Here's how the part is built. I have some questions about the finished solid (model axes, mm). A direction names the side the tool comes from. Round coordinates to 2 decimals unless told otherwise and drop trailing zeros. Order: outer loops, then holes, each group sorted by start corner. A loop starts at its lowest first (then second) coordinate and runs counter-clockwise, first axis right, second up. Notation, with made-up numbers: (60.5, 41.25) -> (89.5, 41.25) arc R23 ccw to (89.5, 63.25) -> close; hole circle Ø11 at (5.5, 36.5). An arc over 180 degrees is marked (long way). Answer in a Markdown table with one row per item.
```python
from build123d import *

# Parameters (mm, degrees)
BOSS_EXTRUDE1_DEPTH     = 35
CUT_EXTRUDE3_DEPTH      = 84.964278119
CUT_EXTRUDE3_DEPTH_BACK = 84.964278119
SKETCH2_R               = 12.5
SKETCH2_R_2             = 15
CUT_EXTRUDE4_START      = 10
CUT_EXTRUDE4_DEPTH      = 25
CHAMFER1_SIZE           = 5


with BuildPart() as part:
    # Sketch1 → Boss-Extrude1 (new body)
    with BuildSketch(Plane(origin=(0, 0, 0), x_dir=(1, 0, 0), z_dir=(0, 1, 0))):
        with BuildLine():
            Line((-40, -16.905989232), (0, -40))
            Line((0, -40), (65, -40))
            Line((65, -40), (65, 20))
            Line((65, 20), (-4.844355629, 20))
            ThreePointArc((-4.844355629, 20), (-38.631222116, 27.900831925), (-40, -6.770509831))
            Line((-40, -6.770509831), (-40, -16.905989232))
        make_face()
    extrude(amount=BOSS_EXTRUDE1_DEPTH)

    # Sketch2 → Cut-Extrude3 (cut, two sides: drawn at the far end of the back side and taken through both)
    with BuildSketch(Plane(origin=(0, 0, 0), x_dir=(1, 0, 0), z_dir=(0, 1, 0)).offset(-CUT_EXTRUDE3_DEPTH_BACK)):
        with Locations(Location((35, -20, 0), (0, 0, 270))):
            Circle(SKETCH2_R)
        with Locations(Location((-25, 10, 0), (0, 0, 270))):
            Circle(SKETCH2_R_2)
    extrude(amount=CUT_EXTRUDE3_DEPTH + CUT_EXTRUDE3_DEPTH_BACK, mode=Mode.SUBTRACT)

    # Sketch3 → Cut-Extrude4 (cut)
    with BuildSketch(Plane(origin=(0, 0, 0), x_dir=(1, 0, 0), z_dir=(0, 1, 0)).offset(CUT_EXTRUDE4_START)):
        Polygon((0, 20), (60, 20), (55, 15), (5, 15), align=None)
        Polygon((65, 10), (65, -30), (60, -25), (60, 5), align=None)
    extrude(amount=CUT_EXTRUDE4_DEPTH, mode=Mode.SUBTRACT)

    # Chamfer1
    chamfer1_edges = [part.edges().sort_by_distance(p)[0] for p in [
        (-20, 35, 28.452994616),
        (-40, 35, 11.838249532),
        (-38.631222116, 35, -27.900831925),
    ]]
    chamfer(chamfer1_edges, length=CHAMFER1_SIZE)


solid = part.part
```
1. Suppose I cut it at A-A on x = 35. Write out the boundary of the cut face in (y, z).
Numbers:
| item | result |
|---|---|
| outline | (0, -20) -> (10, -20) -> (10, -15) -> (35, -15) -> (35, 7.5) -> (0, 7.5) -> close; (0, 32.5) -> (35, 32.5) -> (35, 40) -> (0, 40) -> close |
2. Suppose I cut it at C-C on z = 20. Write out the boundary of the cut face in (x, y).
Numbers:
| item | result |
|---|---|
| outline | (-34.64, 0) -> (22.5, 0) -> (22.5, 35) -> (-24.64, 35) -> (-34.64, 30) -> close; (47.5, 0) -> (65, 0) -> (65, 10) -> (60, 10) -> (60, 35) -> (47.5, 35) -> close |
3. For pin 1 Ø12 at (x, z) = (-22, 21) entering from -Y; pin 2 Ø2 at (x, y) = (24.5, 4.5) entering from -Z; pin 3 Ø8 at (y, z) = (16, 13) entering from -X; pin 4 Ø7.5 at (y, z) = (21.5, 16) entering from +X, each with a flat end and sliding along its axis, tell me the tip position at first contact or that it passes through.
Numbers:
| item | result |
|---|---|
| pin 1 | stops at y = 0 |
| pin 2 | stops at z = -20 |
| pin 3 | stops at x = -40 |
| pin 4 | stops at x = 60 |
4. For faces 1 (the face through (-40, 15, 12)), 2 (the face through (63, 10, 10)), 3 (the face through (-37, 33, 11)), 4 (the face through (3, 22, -17)), which set-ups out of +Z, -Z, +X, -X, +Y, -Y let a thin tool reach every point of the face, with its end or its side?
Numbers:
| item | result |
|---|---|
| face 1 | +Z, -X, +Y, -Y |
| face 2 | +X, +Y |
| face 3 | +Z, -X, +Y |
| face 4 | -Z, +Y |
5. Suppose I cut it at D-D on x = 13. Write out the boundary of the cut face in (y, z), then the cut area to 4 significant figures.
Numbers:
| item | result |
|---|---|
| outline | (0, -20) -> (10, -20) -> (10, -15) -> (35, -15) -> (35, 40) -> (0, 40) -> close |
| area | 1,975 mm2 |
6. We'd pull the mould along Z, two halves only. Please class faces 5 (the face through (-15.315, 32.535, 28.231)), 6 (the face through (8, 0, 11)), 7 (the face through (63, 22, 28)), 8 (the face through (58, 22, -18)): released by +Z, released by -Z, zero draft, split by the parting line, or undercut.
Numbers:
| item | result |
|---|---|
| face 5 | released by +Z |
| face 6 | zero draft |
| face 7 | undercut |
| face 8 | released by -Z |
7. Suppose I cut it at B-B on y = 28.5. Write out the boundary of the cut face in (x, z), then the cut area to 3 significant figures.
Numbers:
| item | result |
|---|---|
| outline | (-40, 6.77) arc R22.5 ccw (long way) to (-4.84, -20) -> (0, -20) -> (5, -15) -> (55, -15) -> (60, -20) -> (65, -20) -> (65, -10) -> (60, -5) -> (60, 25) -> (65, 30) -> (65, 40) -> (0, 40) -> (-40, 16.91) -> close; hole circle Ø30 at (-25, -10); hole circle Ø25 at (35, 20) |
| area | 4,710 mm2 |
8. Please list where these lines run through material, in increasing order: line 1 along X through (y, z) = (19.5, -10); line 2 along Z through (x, y) = (34.5, 26); line 3 along X through (y, z) = (14, 20).
Numbers:
| item | result |
|---|---|
| line 1 | x = -47.5 to -40, -10 to 65 |
| line 2 | z = -15 to 7.51, 32.49 to 40 |
| line 3 | x = -34.64 to 22.5, 47.5 to 60 |
